Source: CAD feature listing. Evaluate the final solid. Frame: model axes, mm. Give positions to 0.01 mm unless a question says otherwise; leave off trailing zeros. Loops run counter-clockwise (first coordinate to the right, second up) from the corner with the lowest first, then second, coordinate; pieces in that order, holes last. Notation, with made-up numbers: M 55.5,56.5 L 108.5,56.5 A20 ccw 108.5,80.5 Z; hole C -14,86.25 d3. An arc over 180 degrees is marked long. Write item = value, one per line.
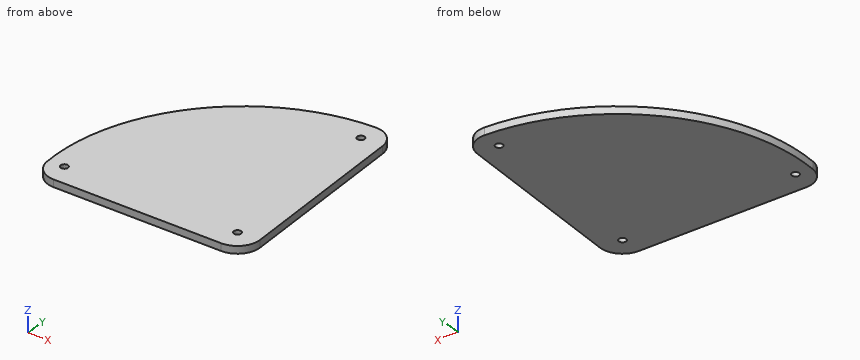
from build123d import *

# Parameters (mm, degrees)
SKETCH_1_R      = 2.5
EXTRUDE_1_DEPTH = 5


with BuildPart() as part:
    # 草图1 → 凸台-拉伸1 (new body)
    with BuildSketch(Plane.XY.offset(-18.206005243)):
        with BuildLine():
            Line((3.867902109, -69.618015729), (120.299999998, -69.618015729))
            ThreePointArc((120.299999998, -69.618015729), (131.246322711, -64.87364925), (135.268196544, -53.641751587))
            Line((135.268196544, -53.641751587), (127.222902207, 69.709644702))
            ThreePointArc((127.222902207, 69.709644702), (122.332732456, 79.843437948), (111.771655863, 83.725600612))
            ThreePointArc((111.771655863, 83.725600612), (20.072255788, 40.438021966), (-11.06192974, -56.06719515))
            ThreePointArc((-11.06192974, -56.06719515), (-6.21332571, -65.725168634), (3.867902109, -69.618015729))
        make_face()
        with Locations(Location((120.299999998, -54.618015744, 0), (0, 0, 180))):
            Circle(SKETCH_1_R, mode=Mode.SUBTRACT)
        with Locations(Location((112.197007482, 69.618015729, 0), (0, 0, 180))):
            Circle(SKETCH_1_R, mode=Mode.SUBTRACT)
        with Locations(Location((0, -54.618015729, 0), (0, 0, 180))):
            Circle(SKETCH_1_R, mode=Mode.SUBTRACT)
    extrude(amount=-EXTRUDE_1_DEPTH)


solid = part.part
1. Cut plane D-D, the plane x = 47.5. Return the cut outline in (y, z).
Derived:
outline = M -69.62,-23.21 L 63.91,-23.21 L 63.91,-18.21 L -69.62,-18.21 Z
2. Cut plane A-A, the plane z = -21.1. Return the cut outline in (x, y).
Derived:
outline = M -11.06,-56.07 A15 ccw 3.87,-69.62 L 120.3,-69.62 A15 ccw 135.27,-53.64 L 127.22,69.71 A15 ccw 111.77,83.73 A127.54 ccw Z; hole C 0,-54.62 d5; hole C 112.2,69.62 d5; hole C 120.3,-54.62 d5
3. Cut plane C-C, the plane y = -6.5. Return the cut outline in (x, z).
Derived:
outline = M -6.1,-23.21 L 132.19,-23.21 L 132.19,-18.21 L -6.1,-18.21 Z
4. Cut plane B-B, the plane x = 0. Return the cut outline in (y, z), then the cut area to 3 significant figures.
Derived:
outline = M -69.11,-23.21 L -57.12,-23.21 L -57.12,-18.21 L -69.11,-18.21 Z; M -52.12,-23.21 L 9.53,-23.21 L 9.53,-18.21 L -52.12,-18.21 Z
area = 368 mm²
5. Material intervals for probe 1 along Y at (x, z) = (120.3, -21.45); probe 2 along Y at (x, z) = (0, -19.9); probe 3 along Y at (x, z) = (18, -22.85), sorted ascending. Write a range as from..to.
Derived:
probe_1 = -69.62..-57.12, -52.12..81.39
probe_2 = -69.11..-57.12, -52.12..9.53
probe_3 = -69.62..38.02
